Could you check a few things on this model? Use its own coordinates, in mm. A direction names the side the tool comes from. Round coordinates to 2 decimals unless told otherwise and drop trailing zeros. Write each loop counter-clockwise with the first axis right and the second up, starting at its lowest first coordinate (ties: lowest second). Pieces come first, ordered by that corner, then holes. Notation, with made-up numbers: (-18.5, -32) -> (-10.5, -32) arc R13 ccw to (-10.5, -25) -> close; hole circle Ø8 at (75.5, -13.75). An arc over 180 degrees is marked (long way). Answer as CSV lines item,"result". Start each with the question number.
Q1. Will these pins go through, and if not, where does the flat tip stop? pin 1 Ø15 at (x, z) = (37.5, 29.5) entering from +Y; pin 2 Ø2 at (x, y) = (46.5, -263.5) entering from +Z.
Q2. If I drill on line 1 (Y direction, x = 36.5, z = 38); line 2 (Z direction, x = 20, y = -215); line 3 (Y direction, x = 54.5, z = 5), over which ranges is the centre line in solid material (lowest first)? Write a range as [from, to].
Q3. If we mould it in two halves opening along Z, with no side actions, what happens to faces 1 (the flat face through (33, -271, 8)), 2 (the flat face through (57.2, -293, 7)), 3 (the flat face through (32, -350, 49))? For each: pulls with the +Z half, pulls with the -Z half, needs draft (parallel to the pull), parting line crosses it, or undercut.
Q4. Imagine slicing it at A-A on y = -234. Please give me the cut outline in (x, z).
Q5. For faces 4 (the cylindrical face through (22.2, -349.9, 43.9)), 5 (the cylindrical face through (55.77, -195.5, 3.94)), 6 (the flat face through (32, -229, 4)), 7 (the flat face through (33, -346, 37)), which set-ups out of +Z, -Z, +X, -X, +Y, -Y let a thin tool reach every point of the face, with its end or its side?
Q6. Imagine slicing it at D-D on x = 44.5. Please give me the cut outline in (y, z).
Q7. Imagine slicing it at B-B on x = 31. Please give me the cut outline in (y, z), and give its area (3 significant figures).
Q8. Imagine slicing it at C-C on z = 44. Please give me the cut outline in (x, y).
from build123d import *

# Parameters (mm, degrees)
PAD002_DEPTH            = 25
POCKET002_DEPTH         = 8.001
POCKET003_DEPTH         = 8.001
FILLET_R                = 5
BODY002_ROLL_ANGLE      = 90
BODY002_PLACEMENT_ANGLE = 90


with BuildPart() as part:
    # Sketch008 → Pad002 (new body, symmetric)
    with BuildSketch(Plane.XY):
        Polygon((0, 0), (0, 80), (8, 80), (8, 8), (160, 8), (160, 0), align=None)
    extrude(amount=PAD002_DEPTH, both=True)

    # Sketch009 (on Face4 of Pad002) → Pocket002 (cut, through all)
    with BuildSketch(Plane(origin=(0, 8, 0), x_dir=(-1, 0, 0), z_dir=(0, 1, 0))):
        with BuildLine():
            ThreePointArc((-115, 5), (-120, 10), (-125, 5))
            Line((-125, 5), (-125, -5))
            ThreePointArc((-125, -5), (-120, -10), (-115, -5))
            Line((-115, 5), (-115, -5))
        make_face()
        with BuildLine():
            ThreePointArc((-53, -5), (-48, -10), (-43, -5))
            Line((-43, -5), (-43, 5))
            ThreePointArc((-43, 5), (-48, 10), (-53, 5))
            Line((-53, -5), (-53, 5))
        make_face()
    extrude(amount=-POCKET002_DEPTH, mode=Mode.SUBTRACT)

    # Sketch010 (on Face15 of Pocket002) → Pocket003 (cut, through all)
    with BuildSketch(Plane.YZ.offset(8)):
        with BuildLine():
            ThreePointArc((39, -5), (44, -10), (49, -5))
            Line((49, -5), (49, 5))
            ThreePointArc((49, 5), (44, 10), (39, 5))
            Line((39, -5), (39, 5))
        make_face()
    extrude(amount=-POCKET003_DEPTH, mode=Mode.SUBTRACT)

    # Fillet
    fillet_edges = [part.edges().sort_by_distance(p)[0] for p in [
        (4, 80, 25),
        (4, 80, -25),
        (160, 4, -25),
        (160, 4, 25),
    ]]
    fillet(fillet_edges, radius=FILLET_R)


with BuildPart() as part_1:
    # Body002 roll: moved
    add(part.part.rotate(Axis((0, 0, 0), (1, 0, 0)), BODY002_ROLL_ANGLE))


with BuildPart() as part_2:
    # Body002 placement: moved
    add(part_1.part.moved(Location((32.2, -354, 0))).rotate(Axis((32.2, -354, 0), (0, 0, 1)), BODY002_PLACEMENT_ANGLE))


solid = part_2.part
Checks:
1,pin 1,"y = -346"
1,pin 2,"z = 8"
2,line 1,"[-354, -346]"
2,line 2,"[0, 8]"
2,line 3,"[-354, -194.56]"
3,face 1,"pulls with the +Z half"
3,face 2,"needs draft"
3,face 3,"undercut"
4,outline,"(7.2, 0) -> (22.2, 0) -> (22.2, 8) -> (7.2, 8) -> close; (42.2, 0) -> (57.2, 0) -> (57.2, 8) -> (42.2, 8) -> close"
5,face 4,"+Y, -Y"
5,face 5,"+Z, -Z, +X, +Y"
5,face 6,"+Z, -Z"
5,face 7,"+Z, +X, -X, +Y"
6,outline,"(-354, 0) -> (-194, 0) -> (-194, 8) -> (-346, 8) -> (-346, 80) -> (-354, 80) -> close"
7,outline,"(-354, 0) -> (-311, 0) -> (-311, 8) -> (-346, 8) -> (-346, 39) -> (-354, 39) -> close; (-354, 49) -> (-346, 49) -> (-346, 80) -> (-354, 80) -> close; (-301, 0) -> (-239, 0) -> (-239, 8) -> (-301, 8) -> close; (-229, 0) -> (-194, 0) -> (-194, 8) -> (-229, 8) -> close"
7,area,"1,620 mm^2"
8,outline,"(7.2, -354) -> (22.2, -354) -> (22.2, -346) -> (7.2, -346) -> close; (42.2, -354) -> (57.2, -354) -> (57.2, -346) -> (42.2, -346) -> close"
